from build123d import *

# Parameters (mm, degrees)
SKETCH1_R           = 8.75
BOSS_EXTRUDE1_DEPTH = 3
BOSS_EXTRUDE2_DEPTH = 10


with BuildPart() as part:
    # Sketch1 → Boss-Extrude1 (new body)
    with BuildSketch(Plane.XY):
        Circle(SKETCH1_R)
    extrude(amount=BOSS_EXTRUDE1_DEPTH)

    # Sketch2 → Boss-Extrude2 (add)
    with BuildSketch(Plane.XY.offset(3)):
        with BuildLine():
            ThreePointArc((4.829991895, 5.737697996), (3.826186326, 5.132311911), (2.976672459, 4.324571779))
            ThreePointArc((2.976672459, 4.324571779), (2.440108702, 4.648480345), (1.868768811, 4.906139331))
            ThreePointArc((1.868768811, 4.906139331), (2.051102492, 6.064099762), (1.979255999, 7.234123699))
            ThreePointArc((1.979255999, 7.234123699), (1.795356309, 7.281943128), (1.610304214, 7.325088418))
            ThreePointArc((1.610304214, 7.325088418), (1.002815466, 6.322553954), (0.62598385, 5.212546807))
            ThreePointArc((0.62598385, 5.212546807), (0.000352422, 5.249999988), (-0.625284028, 5.212630803))
            ThreePointArc((-0.625284028, 5.212630803), (-1.001966616, 6.322688531), (-1.609320762, 7.325304546))
            ThreePointArc((-1.609320762, 7.325304546), (-1.794378647, 7.2821841), (-1.978284756, 7.234389361))
            ThreePointArc((-1.978284756, 7.234389361), (-2.050288332, 6.06437508), (-1.868110115, 4.90639018))
            ThreePointArc((-1.868110115, 4.90639018), (-2.439484593, 4.648807903), (-2.976091832, 4.324971377))
            ThreePointArc((-2.976091832, 4.324971377), (-3.825497247, 5.132825554), (-4.82922153, 5.738346401))
            ThreePointArc((-4.82922153, 5.738346401), (-4.97304308, 5.614164455), (-5.113672529, 5.486378884))
            ThreePointArc((-5.113672529, 5.486378884), (-4.633695781, 4.41692096), (-3.934242565, 3.476238691))
            ThreePointArc((-3.934242565, 3.476238691), (-4.320465088, 2.982629951), (-4.645112863, 2.44651313))
            ThreePointArc((-4.645112863, 2.44651313), (-5.772652562, 2.7670941), (-6.942805845, 2.83680225))
            ThreePointArc((-6.942805845, 2.83680225), (-7.012443275, 2.66000739), (-7.077579552, 2.481505124))
            ThreePointArc((-7.077579552, 2.481505124), (-6.15557937, 1.757603477), (-5.099087457, 1.249722811))
            ThreePointArc((-5.099087457, 1.249722811), (-5.211679097, 0.633167423), (-5.249994516, 0.007588209))
            ThreePointArc((-5.249994516, 0.007588209), (-6.397362742, -0.232545265), (-7.46587701, -0.71461911))
            ThreePointArc((-7.46587701, -0.71461911), (-7.445377224, -0.90352531), (-7.420098394, -1.091851556))
            ThreePointArc((-7.420098394, -1.091851556), (-6.267293907, -1.304359781), (-5.095792863, -1.263089504))
            ThreePointArc((-5.095792863, -1.263089504), (-4.908960234, -1.861346132), (-4.652165695, -2.43307508))
            ThreePointArc((-4.652165695, -2.43307508), (-5.556514215, -3.178911313), (-6.278605726, -4.102329843))
            ThreePointArc((-6.278605726, -4.102329843), (-6.172664978, -4.260071251), (-6.062762116, -4.415078202))
            ThreePointArc((-6.062762116, -4.415078202), (-4.94324694, -4.067509932), (-3.925113535, -3.486543236))
            ThreePointArc((-3.925113535, -3.486543236), (-3.48165774, -3.92944772), (-2.988581778, -4.316350189))
            ThreePointArc((-2.988581778, -4.316350189), (-3.442735244, -5.397027088), (-3.652981535, -6.550246247))
            ThreePointArc((-3.652981535, -6.550246247), (-3.485869574, -6.640686208), (-3.316520101, -6.726863639))
            ThreePointArc((-3.316520101, -6.726863639), (-2.486761671, -5.898842577), (-1.855237999, -4.91127193))
            ThreePointArc((-1.855237999, -4.91127193), (-1.256749416, -5.09736019), (-0.640349792, -5.210801488))
            ThreePointArc((-0.640349792, -5.210801488), (-0.540267119, -6.378748999), (-0.190503298, -7.497580176))
            ThreePointArc((-0.190503298, -7.497580176), (-0.00050346, -7.499999983), (0.189496701, -7.497605685))
            ThreePointArc((0.189496701, -7.497605685), (0.539410728, -6.378821476), (0.639650205, -5.210887412))
            ThreePointArc((0.639650205, -5.210887412), (1.256065053, -5.09752887), (1.854578614, -4.911520962))
            ThreePointArc((1.854578614, -4.911520962), (2.485969693, -5.899176387), (3.315616949, -6.727308842))
            ThreePointArc((3.315616949, -6.727308842), (3.48497799, -6.641154147), (3.652102092, -6.550736623))
            ThreePointArc((3.652102092, -6.550736623), (3.44201063, -5.397489248), (2.988002255, -4.316751385))
            ThreePointArc((2.988002255, -4.316751385), (3.481130156, -3.929915118), (3.92464541, -3.487070175))
            ThreePointArc((3.92464541, -3.487070175), (4.942700807, -4.068173557), (6.06216931, -4.415892125))
            ThreePointArc((6.06216931, -4.415892125), (6.172092982, -4.260899931), (6.278054907, -4.103172747))
            ThreePointArc((6.278054907, -4.103172747), (5.556087377, -3.17965728), (4.651838998, -2.433699639))
            ThreePointArc((4.651838998, -2.433699639), (4.908710292, -1.862005173), (5.09562324, -1.263773634))
            ThreePointArc((5.09562324, -1.263773634), (6.267118732, -1.305201192), (7.41995174, -1.092847739))
            ThreePointArc((7.41995174, -1.092847739), (7.445255854, -0.904524889), (7.465781001, -0.715621443))
            ThreePointArc((7.465781001, -0.715621443), (6.397331464, -0.233404148), (5.249995488, 0.006883365))
            ThreePointArc((5.249995488, 0.006883365), (5.211764057, 0.632467717), (5.099255194, 1.249038216))
            ThreePointArc((5.099255194, 1.249038216), (6.155815283, 1.756777037), (7.077912646, 2.480554893))
            ThreePointArc((7.077912646, 2.480554893), (7.012800334, 2.659065903), (6.94318664, 2.83587011))
            ThreePointArc((6.94318664, 2.83587011), (5.773024009, 2.766319061), (4.64544128, 2.445889473))
            ThreePointArc((4.64544128, 2.445889473), (4.320865485, 2.982049876), (3.934709236, 3.475710464))
            ThreePointArc((3.934709236, 3.475710464), (4.634288738, 4.416298818), (5.114409063, 5.485692293))
            ThreePointArc((5.114409063, 5.485692293), (4.973796771, 5.613496743), (4.829991895, 5.737697996))
        make_face()
    extrude(amount=BOSS_EXTRUDE2_DEPTH)


solid = part.part
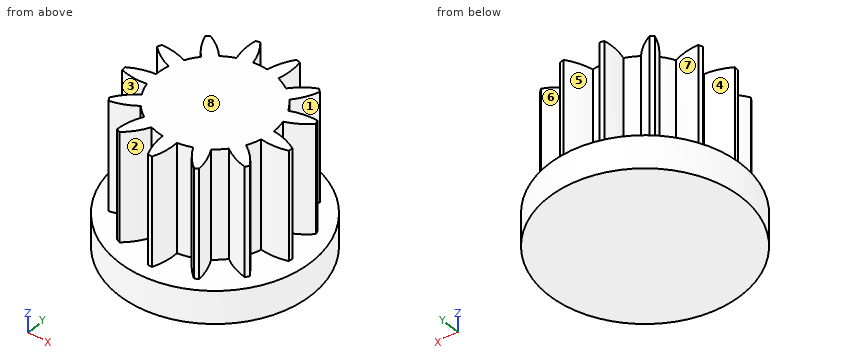
The listing builds one solid part. Answer for the finished solid, in the listing's coordinates (mm). Face numbers are marked on the shaded views. A direction names the side the tool comes from. Round coordinates to 2 decimals unless told otherwise and drop trailing zeros. Write each loop counter-clockwise with the first axis right and the second up, starting at its lowest first coordinate (ties: lowest second). Pieces come first, ordered by that corner, then holes. Notation, with made-up numbers: M 2.5,2.25 L 18.5,2.25 A17 cw 18.5,9.25 Z; hole C 13,-3.75 d2. An arc over 180 degrees is marked long. Write each question's results on one line, items separated by ' | '. Start each with the question number.
(1) Each of these flat-tipped pins is pushed along its axis until it touches: P1, Ø5, axis at x = 2.5, z = 11, coming from the -Y side; P2, Ø1.5, axis at x = -5, z = 4.5, coming from the +Y side; P3, Ø5, axis at y = 1, z = 6.5, coming from the +X side; P4, Ø2, axis at x = 7, y = 1.5, coming from the +Z side. Where does it stop, or does it pass through?
(2) Determine the mould class of the marked faces 6, 7 and 8 for opening direction Y: +Y half, -Y half, draft (parallel to the pull), parting line (faces both ways), or undercut.
(3) Find the intervals of material crossed by line 1 (Z direction, x = -4, y = -5); line 2 (Y direction, x = -6.75, z = 7.75); line 3 (X direction, y = 5, z = 11), in increasing order.
(4) The part is cut by section A-A, the plane y = -6. Write down the section's boundary in (x, z) (3 decimals), and give its area (3 significant figures).
(5) For the marked faces 1, 2, 3, 4 and 5, determine the directions among +Z, -Z, +X, -X, +Y, -Y from which every point of the face is accessible in a straight line to the end or side of a thin tool.
(6) The part is cut by section B-B, the plane x = 1. Write down the section's boundary in (y, z), and give its area (3 significant figures).
Worked answers:
1) P1: stops at y = -7.5 | P2: stops at y = 5.74 | P3: stops at x = 7.47 | P4: stops at z = 13
2) face 6: +Y half | face 7: undercut | face 8: draft
3) line 1: z = 0 to 3 | line 2: y = -1.25 to -0.36, 2.19 to 2.84 | line 3: x = -4.93 to -3.66, -1.89 to 1.89, 3.66 to 4.93
4) outline: M -6.369,0 L 6.369,0 L 6.369,3 L 3.584,3 L 3.584,13 L 2.569,13 L 2.569,3 L 0.6,3 L 0.6,13 L -0.601,13 L -0.601,3 L -2.57,3 L -2.57,13 L -3.585,13 L -3.585,3 L -6.369,3 Z | area: 70.5 mm²
5) face 1: +Z, +X | face 2: +Z, -Y | face 3: +Z | face 4: +Z, -X | face 5: +Z, +Y
6) outline: M -8.69,0 L 8.69,0 L 8.69,3 L 6.32,3 L 6.32,13 L -5.15,13 L -5.15,3 L -8.69,3 Z | area: 167 mm²
